Model file for the job. Use its own axes, mm. Round coordinates to 2 decimals unless told otherwise and drop trailing zeros. Order: outer loops, then holes, each group sorted by start corner. A loop starts at its lowest first (then second) coordinate and runs counter-clockwise, first axis right, second up. Notation, with made-up numbers: (-9.75, 9) - (40.25, 9) arc R24 ccw to (40.25, 27) - close; hole circle Ø3 at (-8.5, 10.5). An arc over 180 degrees is marked (long way). Answer as CSV lines item,"result". Start each with the question number.
1. Band-saw the part on C-C on y = -2.2. List the corners of the cut face in (x, z) (3 decimals).
2. Band-saw the part on A-A on x = -25.5. List the corners of the cut face in (y, z) (3 decimals), then the cut area to 4 significant figures.
3. Pin check, flat tip, straight feed: pin 1 Ø5.5 at (x, z) = (-25.5, 0) entering from -Y. Stop position of the tip, or through.
4. Band-saw the part on D-D on x = -35. List the corners of the cut face in (y, z).
5. Pull direction X, two halves, no side cores. Call faces 1 (the face through (33.61, -0.49, 6.44)), 2 (the face through (-40, -1, 0)), 3 (the face through (22.13, -1.48, 0.15)), 4 (the face through (-1, -1, -12.5)): released by +X, released by -X, zero draft, split by the parting line, or undercut.
6. Wall check: line 1 along Z through (x, y) = (35, -0.75); line 2 along Z through (x, y) = (-25.5, -2.15) (3 decimals); line 3 along X through (y, z) = (-2.35, 9.5). Give the ranges that are in metal, low to high. Write a range as [from, to].
7. Band-saw the part on B-B on z = 7.5. List the corners of the cut face in (x, y).
```python
from build123d import *

# Parameters (mm, degrees)
F0_W     = 80
F0_H     = 25
F0_R     = 1.75
F0_R_2   = 3.375
F1_DEPTH = 3
F2_SIZE  = 2


with BuildPart() as f1:
    # F0 (on Front) → F1 (new body)
    with BuildSketch(Plane.XZ):
        Rectangle(F0_W, F0_H)
        with Locations((0, -7.5)):
            Circle(F0_R, mode=Mode.SUBTRACT)
        with Locations((-25.5, 0)):
            Circle(F0_R_2, mode=Mode.SUBTRACT)
        with Locations((-35, 7.5)):
            Circle(F0_R, mode=Mode.SUBTRACT)
        with Locations((25.5, 0)):
            Circle(F0_R_2, mode=Mode.SUBTRACT)
        with Locations((35, 7.5)):
            Circle(F0_R, mode=Mode.SUBTRACT)
    extrude(amount=F1_DEPTH)

    # F2
    f2_edges = [f1.edges().sort_by_distance(p)[0] for p in [
        (-36.75, -3, 7.5),
        (-1.75, -3, -7.5),
        (33.25, -3, 7.5),
    ]]
    chamfer(f2_edges, length=F2_SIZE)


solid = f1.part
```
Reply:
1,outline,"(-40, -12.5) - (40, -12.5) - (40, 12.5) - (-40, 12.5) - close; hole circle Ø5.9 at (-35, 7.5); hole circle Ø6.75 at (-25.5, 0); hole circle Ø5.9 at (0, -7.5); hole circle Ø6.75 at (25.5, 0); hole circle Ø5.9 at (35, 7.5)"
2,outline,"(-3, -12.5) - (0, -12.5) - (0, -3.375) - (-3, -3.375) - close; (-3, 3.375) - (0, 3.375) - (0, 12.5) - (-3, 12.5) - close"
2,area,"54.75 mm2"
3,pin 1,"passes through"
4,outline,"(-3, -12.5) - (0, -12.5) - (0, 5.75) - (-1, 5.75) - (-3, 3.75) - close; (-3, 11.25) - (-1, 9.25) - (0, 9.25) - (0, 12.5) - (-3, 12.5) - close"
5,face 1,"undercut"
5,face 2,"released by -X"
5,face 3,"undercut"
5,face 4,"zero draft"
6,line 1,"z = [-12.5, 5.75], [9.25, 12.5]"
6,line 2,"z = [-12.5, -3.375], [3.375, 12.5]"
6,line 3,"x = [-40, -37.37], [-32.63, 32.63], [37.37, 40]"
7,outline,"(-40, -3) - (-38.75, -3) - (-36.75, -1) - (-36.75, 0) - (-40, 0) - close; (-33.25, -1) - (-31.25, -3) - (31.25, -3) - (33.25, -1) - (33.25, 0) - (-33.25, 0) - close; (36.75, -1) - (38.75, -3) - (40, -3) - (40, 0) - (36.75, 0) - close"
